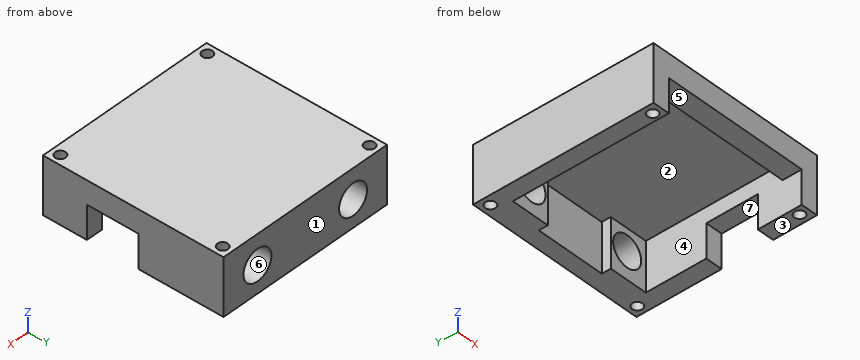
```python
from build123d import *

# Parameters (mm, degrees)
SKETCH_1_W          = 70.091778518
SKETCH_1_H          = 70.091778518
SKETCH_1_R          = 2
EXTRUDE_1_DEPTH     = 22
CUT_EXTRUDE_4_DEPTH = 19
SKETCH_4_R          = 6
CUT_EXTRUDE_5_DEPTH = 15
SKETCH_4_3_R        = 6
CUT_EXTRUDE_6_DEPTH = 15
SKETCH_5_W          = 13
SKETCH_5_H          = 20
CUT_EXTRUDE_7_DEPTH = 10
SKETCH_6_W          = 57
SKETCH_6_H          = 13
CUT_EXTRUDE_8_DEPTH = 16


with BuildPart() as part:
    # Sketch 1 → Extrude 1 (new body)
    with BuildSketch(Plane.XY):
        Rectangle(SKETCH_1_W, SKETCH_1_H)
        with Locations((-31.5, -31.5)):
            Circle(SKETCH_1_R, mode=Mode.SUBTRACT)
        with Locations((-31.5, 31.5)):
            Circle(SKETCH_1_R, mode=Mode.SUBTRACT)
        with Locations((31.5, 31.5)):
            Circle(SKETCH_1_R, mode=Mode.SUBTRACT)
        with Locations((31.5, -31.5)):
            Circle(SKETCH_1_R, mode=Mode.SUBTRACT)
    extrude(amount=EXTRUDE_1_DEPTH)

    # Sketch 2 → Cut-Extrude 4 (cut)
    with BuildSketch(Plane.XY):
        Polygon((-28.5, 25.5), (-13.5, 25.5), (-13.5, 29), (13.5, 29), (13.5, 25.5), (28.5, 25.5), (28.5, -27.6), (-28.5, -27.6), align=None)
    extrude(amount=CUT_EXTRUDE_4_DEPTH, mode=Mode.SUBTRACT)

    # Sketch 4 → Cut-Extrude 5 (cut)
    with BuildSketch(Plane(origin=(0, 35.045889259, 0), x_dir=(1, 0, 0), z_dir=(0, 1, 0))):
        with Locations(Location((20.5, -10.5, 0), (0, 0, 270))):
            Circle(SKETCH_4_R)
    extrude(amount=-CUT_EXTRUDE_5_DEPTH, mode=Mode.SUBTRACT)

    # Sketch 4_3 → Cut-Extrude 6 (cut)
    with BuildSketch(Plane(origin=(0, 35.045889259, 0), x_dir=(1, 0, 0), z_dir=(0, 1, 0))):
        with Locations(Location((20.5, -10.5, 0), (0, 0, 270))):
            Circle(SKETCH_4_3_R)
        with Locations(Location((-20.5, -10.5, 0), (0, 0, 270))):
            Circle(SKETCH_4_3_R)
    extrude(amount=-CUT_EXTRUDE_6_DEPTH, mode=Mode.SUBTRACT)

    # Sketch 5 → Cut-Extrude 7 (cut)
    with BuildSketch(Plane(origin=(35.045889259, 0, 0), x_dir=(0, 0, -1), z_dir=(1, 0, 0))):
        with Locations((-6.5, -8)):
            Rectangle(SKETCH_5_W, SKETCH_5_H)
    extrude(amount=-CUT_EXTRUDE_7_DEPTH, mode=Mode.SUBTRACT)

    # Sketch 6 → Cut-Extrude 8 (cut)
    with BuildSketch(Plane(origin=(0, -35.045889259, 0), x_dir=(-1, 0, 0), z_dir=(0, -1, 0))):
        with Locations((0, -6.5)):
            Rectangle(SKETCH_6_W, SKETCH_6_H)
    extrude(amount=-CUT_EXTRUDE_8_DEPTH, mode=Mode.SUBTRACT)


solid = part.part
```
Geometry: final body of the model. Coordinates: model frame, mm. Face numbers are marked on the shaded views. A direction names the side the tool comes from. Coordinates: 2 decimals unless noted, no trailing zeros. Order: outer loops, then holes, each group sorted by start corner. A loop starts at its lowest first (then second) coordinate and runs counter-clockwise, first axis right, second up. Notation, with made-up numbers: (77, -40) -> (102, -40) arc R13 ccw to (102, -19) -> close; hole circle Ø9 at (-33.5, -26.75). An arc over 180 degrees is marked (long way). Write each question's results on one line, items separated by ' | '. Start each with the question number.
1) Cut plane D-D, the plane y = -31.5. Output: boundary loops of the cut face in (x, z).
2) Material intervals for line 1 along Y through (x, z) = (31.5, 7); line 2 along Y through (x, z) = (-31.5, 8.75); line 3 along X through (y, z) = (24, 14), sorted ascending.
3) First-contact query: pin 1 (2 mm diameter, centred on x = 8.5, y = -32.5, fed in from -Z); pin 2 (1.5 mm diameter, centred on y = -10, z = 3, fed in from +X); pin 3 (11 mm diameter, centred on x = 20.5, z = 10.5, fed in from +Y). Flat tips, straight axial feed; report the tip coordinate or a pass-through.
4) Set-up query: the marked faces 4, 5, 6 and 7. Return all of +Z, -Z, +X, -X, +Y, -Y with unobstructed straight access to the full face (end or side cutting, diameter ignored); none if empty.
5) Cut plane C-C, the plane x = 20.5. Output: boundary loops of the cut face in (y, z).
6) Cut plane B-B, the plane z = 2.5. Output: boundary loops of the cut face in (x, y), and give its area (3 significant figures).
7) Mould query, pull axis Y, two halves, no side actions, for the marked faces 1, 2 and 3. Classes: released by +Y, released by -Y, zero draft, split by the parting line, or undercut.
8) Cut plane A-A, the plane y = 31.5. Output: boundary loops of the cut face in (x, z).
Checks:
1) outline: (-35.05, 0) -> (-33.5, 0) -> (-33.5, 22) -> (-35.05, 22) -> close; (-29.5, 0) -> (-28.5, 0) -> (-28.5, 13) -> (28.5, 13) -> (28.5, 0) -> (29.5, 0) -> (29.5, 22) -> (-29.5, 22) -> close; (33.5, 0) -> (35.05, 0) -> (35.05, 22) -> (33.5, 22) -> close
2) line 1: -35.05 to -33.5, -29.5 to -18, 2 to 29.5, 33.5 to 35.05 | line 2: -35.05 to -33.5, -29.5 to 29.5, 33.5 to 35.05 | line 3: -35.05 to -28.5, 28.5 to 35.05
3) pin 1: z = 13 | pin 2: x = -28.5 | pin 3: y = -27.6
4) face 4: -Z | face 5: -Z, -Y | face 6: +Y | face 7: -Z, +X
5) outline: (-35.05, 13) -> (-27.6, 13) -> (-27.6, 19) -> (25.5, 19) -> (25.5, 16.5) -> (35.05, 16.5) -> (35.05, 22) -> (-35.05, 22) -> close; (25.5, 0) -> (35.05, 0) -> (35.05, 4.5) -> (25.5, 4.5) -> close
6) outline: (-35.05, -35.05) -> (-28.5, -35.05) -> (-28.5, 25.5) -> (-13.5, 25.5) -> (-13.5, 29) -> (13.5, 29) -> (13.5, 25.5) -> (28.5, 25.5) -> (28.5, 2) -> (35.05, 2) -> (35.05, 35.05) -> (-35.05, 35.05) -> close; (28.5, -35.05) -> (35.05, -35.05) -> (35.05, -18) -> (28.5, -18) -> close; hole circle Ø4 at (-31.5, -31.5); hole circle Ø4 at (-31.5, 31.5); hole circle Ø4 at (31.5, -31.5); hole circle Ø4 at (31.5, 31.5) | area: 1,190 mm^2
7) face 1: released by +Y | face 2: undercut | face 3: zero draft
8) outline: (-35.05, 0) -> (-33.5, 0) -> (-33.5, 22) -> (-35.05, 22) -> close; (-29.5, 0) -> (29.5, 0) -> (29.5, 22) -> (-29.5, 22) -> close; (33.5, 0) -> (35.05, 0) -> (35.05, 22) -> (33.5, 22) -> close; hole circle Ø12 at (-20.5, 10.5); hole circle Ø12 at (20.5, 10.5)
